Read the model definition and answer for the solid it produces. Units are mm, in the model's axes. A direction names the side the tool comes from. Round coordinates to 2 decimals unless told otherwise and drop trailing zeros. Order: outer loops, then holes, each group sorted by start corner. A loop starts at its lowest first (then second) coordinate and runs counter-clockwise, first axis right, second up.
from build123d import *

# Parameters (mm, degrees)
CROQUIS1_W              = 70
CROQUIS1_H              = 70
CROQUIS1_R              = 4
SALIENTE_EXTRUIR1_DEPTH = 12
CROQUIS3_R              = 4
CORTAR_EXTRUIR2_DEPTH   = 15
CROQUIS4_W              = 40
CROQUIS4_H              = 15
SALIENTE_EXTRUIR2_DEPTH = 12
CROQUIS6_R              = 4
CORTAR_EXTRUIR4_DEPTH   = 15


with BuildPart() as part:
    # Croquis1 → Saliente-Extruir1 (new body)
    with BuildSketch(Plane(origin=(0, 0, 0), x_dir=(1, 0, 0), z_dir=(0, 1, 0))):
        Rectangle(CROQUIS1_W, CROQUIS1_H)
        Circle(CROQUIS1_R, mode=Mode.SUBTRACT)
    extrude(amount=SALIENTE_EXTRUIR1_DEPTH)

    # Croquis3 → Cortar-Extruir2 (cut)
    with BuildSketch(Plane(origin=(0, 12, 0), x_dir=(1, 0, 0), z_dir=(0, 1, 0))):
        with Locations((-28, 14)):
            Circle(CROQUIS3_R)
        with Locations((28, 14)):
            Circle(CROQUIS3_R)
        with Locations((28, -14)):
            Circle(CROQUIS3_R)
        with Locations((-28, -14)):
            Circle(CROQUIS3_R)
    extrude(amount=-CORTAR_EXTRUIR2_DEPTH, mode=Mode.SUBTRACT)

    # Croquis4 → Saliente-Extruir2 (add)
    with BuildSketch(Plane(origin=(0, 12, 0), x_dir=(1, 0, 0), z_dir=(0, 1, 0))):
        with Locations((-35, 0)):
            Rectangle(CROQUIS4_W, CROQUIS4_H)
    extrude(amount=-SALIENTE_EXTRUIR2_DEPTH)

    # Croquis6 → Cortar-Extruir4 (cut)
    with BuildSketch(Plane.XY.offset(7.5)):
        with Locations((-45, 6)):
            Circle(CROQUIS6_R)
    extrude(amount=-CORTAR_EXTRUIR4_DEPTH, mode=Mode.SUBTRACT)


solid = part.part
Q1. A cutting plane is placed at D-D, the plane z = -14. Give the vertices of the cut face in (x, y), plus the area to 3 significant figures.
Outcome:
outline: (-35, 0) - (-32, 0) - (-32, 12) - (-35, 12) - close; (-24, 0) - (24, 0) - (24, 12) - (-24, 12) - close; (32, 0) - (35, 0) - (35, 12) - (32, 12) - close
area: 648 mm2
Q2. A cutting plane is placed at C-C, the plane x = 28. Give the vertices of the cut face in (y, z), plus the area to 3 significant figures.
Outcome:
outline: (0, -35) - (12, -35) - (12, -18) - (0, -18) - close; (0, -10) - (12, -10) - (12, 10) - (0, 10) - close; (0, 18) - (12, 18) - (12, 35) - (0, 35) - close
area: 648 mm2
Q3. For faces 4 (the face through (25.05, 6.08, -16.7)), 5 (the face through (-50, 6, -7.5)), 6 (the face through (-50, 6, 7.5)), determine the directions among +Z, -Z, +X, -X, +Y, -Y from which every point of the face is accessible in a straight line to the end or side of a thin tool.
Outcome:
face 4: +Y, -Y
face 5: -Z, -X, +Y, -Y
face 6: +Z, -X, +Y, -Y
Q4. A cutting plane is placed at A-A, the plane y = 6. Give the vertices of the cut face in (x, z), plus the area to 3 significant figures.
Outcome:
outline: (-55, -7.5) - (-49, -7.5) - (-49, 7.5) - (-55, 7.5) - close; (-41, -7.5) - (-35, -7.5) - (-35, -35) - (35, -35) - (35, 35) - (-35, 35) - (-35, 7.5) - (-41, 7.5) - close; hole circle Ø8 at (-28, -14); hole circle Ø8 at (-28, 14); hole circle Ø8 at (0, 0); hole circle Ø8 at (28, -14); hole circle Ø8 at (28, 14)
area: 4,830 mm2
Q5. Straight lines are drawn through the part: probe 1 along X at (y, z) = (4.25, -14); probe 2 along Z at (x, y) = (-28, 6.5); probe 3 along Z at (x, y) = (0, 6). For each, find the intervals that lie inside material, in ascending order.
Outcome:
probe 1: x = -35 to -32, -24 to 24, 32 to 35
probe 2: z = -35 to -18, -10 to 10, 18 to 35
probe 3: z = -35 to -4, 4 to 35
Q6. Flat-ended cylindrical pins translate along their axes: pin 1 (6 mm diameter, centred on x = -40.5, y = 8.5, fed in from +Z); pin 2 (9 mm diameter, centred on x = 28, z = 14, fed in from -Y); pin 3 (3.5 mm diameter, centred on x = -48.5, y = 6.5, fed in from -Z); pin 4 (3.5 mm diameter, centred on y = 9, z = -26.5, fed in from -X). Find the tip coordinate at first contact, or state that the pin passes through.
Outcome:
pin 1: stops at z = 7.5
pin 2: stops at y = 0
pin 3: stops at z = -7.5
pin 4: stops at x = -35
Q7. A cutting plane is placed at B-B, the plane z = 0. Give the vertices of the cut face in (x, y).
Outcome:
outline: (-55, 0) - (-4, 0) - (-4, 12) - (-55, 12) - close; (4, 0) - (35, 0) - (35, 12) - (4, 12) - close; hole circle Ø8 at (-45, 6)
Q8. For a pull along Y with two mould halves and no side action, classify faces 1 (the face through (-48.2, 3.6, 0.1)), 2 (the face through (-55, 6, 0)), 3 (the face through (-11, 12, 0)) as released by +Y, released by -Y, zero draft, split by the parting line, or undercut.
Outcome:
face 1: undercut
face 2: zero draft
face 3: released by +Y
